The figure shows three views and two pictorial views of one solid part (mm, origin at its lowest corner). Answer the questions. A direction names the side the tool comes from. Coordinates: 2 decimals unless noted, no trailing zeros. Write each loop counter-clockwise with the first axis right and the second up, starting at its lowest first coordinate (ties: lowest second). Pieces come first, ordered by that corner, then holes. Notation, with made-up numbers: (54.25, 37.25) - (93.25, 37.25) arc R8 ccw to (93.25, 50.25) - close; hole circle Ø3 at (-19, -31.75). An arc over 180 degrees is marked (long way). Use a Markdown table: item, result. Add a question column.
(1) The part is cut by section B-B, the plane x = 30. Give the vertices of the cut face in (y, z), then the cut area to 4 significant figures.
(2) A tool of negligible diameter and unlimited length cuts with its end or side. For the marked faces 1, 2 and 3, from which of +Z, -Z, +X, -X, +Y, -Y can it reach the whole face along a straight path? Write none if from no direction.
(3) Given pin 1 Ø10 at (y, z) = (9.5, 39) entering from -X; pin 2 Ø2.5 at (x, z) = (65, 44.5) entering from -Y (3 decimals); pin 3 Ø20 at (y, z) = (22, 20) entering from +X; pin 4 Ø9 at (x, z) = (10, 10) entering from -Y, each flat-ended and moving along its own axis, determine where each tip first touches the part or whether it passes through.
(4) Find the intervals of material crossed by line 1 (Z direction, x = 65, y = 1); line 2 (Z direction, x = 10, y = 33.7); line 3 (Y direction, x = 37, z = 12.5), in increasing order. Write a range as from..to.
(5) The part is cut by section A-A, the plane z = 30. Give the vertices of the cut face in (x, y), then the cut area to 4 significant figures.
(6) The part is cut by section C-C, the plane y = 32.5. Give the vertices of the cut face in (x, z).
(7) The part is cut by section D-D, the plane z = 50. Give the vertices of the cut face in (x, y).
(8) For a pull along Y with two mould halves and no side action, classify the marked faces 4, 5 and 6 as released by +Y, released by -Y, zero draft, split by the parting line, or undercut.
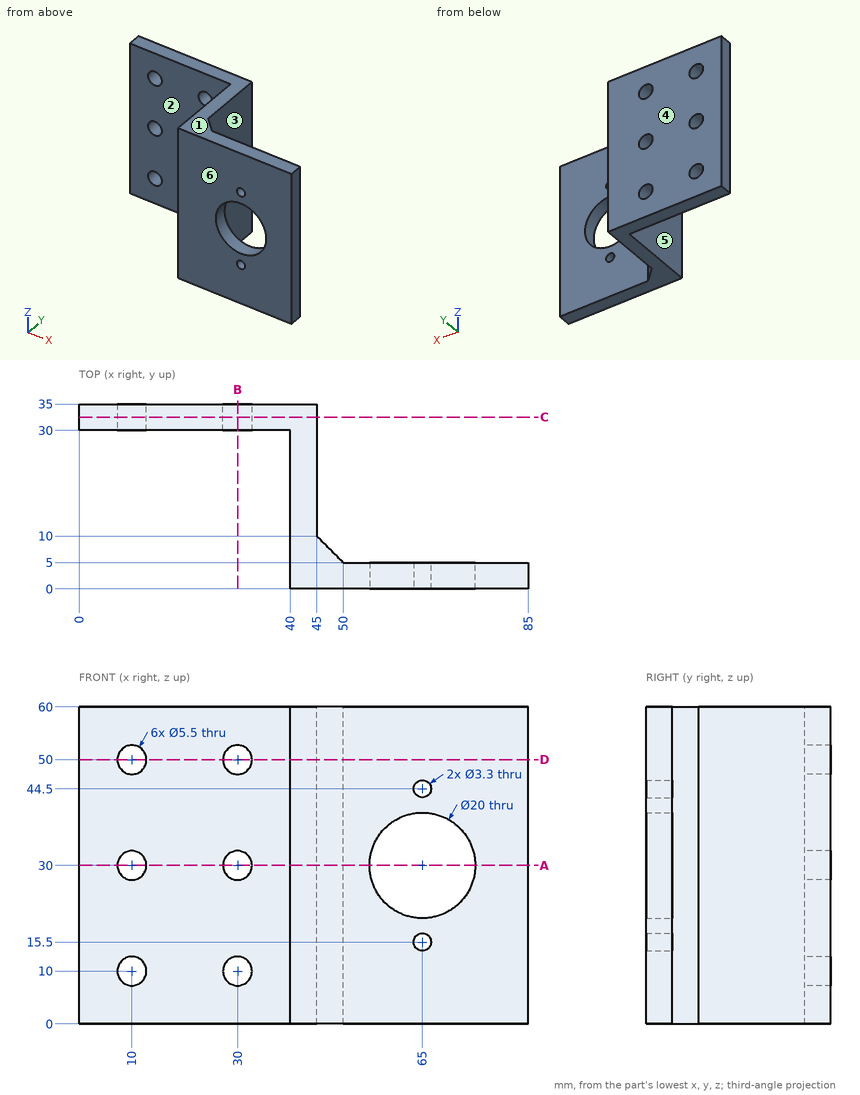
Model answer:
| question | item | result |
|---|---|---|
| 1 | outline | (30, 0) - (35, 0) - (35, 7.25) - (30, 7.25) - close; (30, 12.75) - (35, 12.75) - (35, 27.25) - (30, 27.25) - close; (30, 32.75) - (35, 32.75) - (35, 47.25) - (30, 47.25) - close; (30, 52.75) - (35, 52.75) - (35, 60) - (30, 60) - close |
| 1 | area | 217.5 mm^2 |
| 2 | face 1 | +Z, +X, -X, +Y, -Y |
| 2 | face 2 | +Z, -Z, -X, -Y |
| 2 | face 3 | +Z, -Z, +X, +Y |
| 3 | pin 1 | x = 40 |
| 3 | pin 2 | through |
| 3 | pin 3 | x = 45 |
| 3 | pin 4 | y = 30 |
| 4 | line 1 | 0..13.85, 17.15..20, 40..42.85, 46.15..60 |
| 4 | line 2 | 0..7.25, 12.75..27.25, 32.75..47.25, 52.75..60 |
| 4 | line 3 | 30..35 |
| 5 | outline | (0, 30) - (7.25, 30) - (7.25, 35) - (0, 35) - close; (12.75, 30) - (27.25, 30) - (27.25, 35) - (12.75, 35) - close; (32.75, 30) - (40, 30) - (40, 0) - (55, 0) - (55, 5) - (50, 5) - (45, 10) - (45, 35) - (32.75, 35) - close; (75, 0) - (85, 0) - (85, 5) - (75, 5) - close |
| 5 | area | 432.5 mm^2 |
| 6 | outline | (0, 0) - (45, 0) - (45, 60) - (0, 60) - close; hole circle Ø5.5 at (10, 10); hole circle Ø5.5 at (10, 30); hole circle Ø5.5 at (10, 50); hole circle Ø5.5 at (30, 10); hole circle Ø5.5 at (30, 30); hole circle Ø5.5 at (30, 50) |
| 7 | outline | (0, 30) - (7.25, 30) - (7.25, 35) - (0, 35) - close; (12.75, 30) - (27.25, 30) - (27.25, 35) - (12.75, 35) - close; (32.75, 30) - (40, 30) - (40, 0) - (85, 0) - (85, 5) - (50, 5) - (45, 10) - (45, 35) - (32.75, 35) - close |
| 8 | face 4 | released by +Y |
| 8 | face 5 | zero draft |
| 8 | face 6 | released by -Y |
